Source: three-view drawing plus pictorial views. Frame: mm from the lowest corner of the part. A direction names the side the tool comes from. Give positions to 0.01 mm unless a question says otherwise; leave off trailing zeros. Write each loop counter-clockwise with the first axis right and the second up, starting at its lowest first coordinate (ties: lowest second). Pieces come first, ordered by that corner, then holes.
Q1. Reachability of the marked faces 1 and 2 from +Z, -Z, +X, -X, +Y, -Y: full face, straight path, thin tool, end or side. Return the list, or none.
Q2. Pin query (flat end, axial travel): pin 1 (1 mm diameter, centred on x = 12, z = 11, fed in from -Y); pin 2 (8 mm diameter, centred on x = 16.5, y = 26.5, fed in from +Z). Return the tip coordinate at first contact, or that it passes through.
Q3. Line query: L1, parallel to X at y = 20.5, z = 10.25; L2, parallel to Y at x = 25, z = 1.5; L3, parallel to Z at x = 10.5, y = 47. Output: solid intervals per line, ascending.
Q4. Cut plane D-D on z = 14.5. Return the cut outline in (x, y), plus the area to 3 significant figures.
Q5. Cut plane A-A on y = 9. Return the cut outline in (x, z).
Q6. Draft query along Y for the marked faces 3, 4 and 5. Return one class per face: pulls with the +Y half, pulls with the -Y half, needs draft (parallel to the pull), parting line crosses it, or undercut.
Q7. Cut plane C-C on y = 37. Return the cut outline in (x, z), plus the area to 3 significant figures.
Q8. Cut plane B-B on x = 41. Return the cut outline in (y, z), plus the area to 3 significant figures.
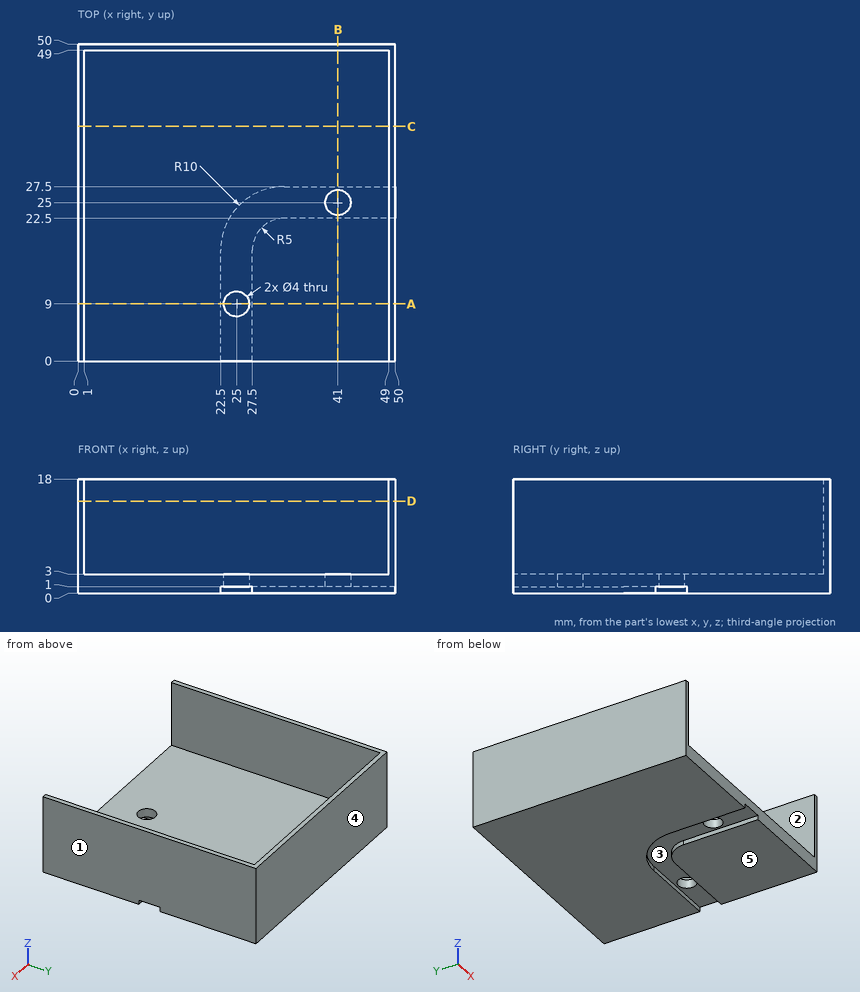
Data:
1. face 1: +Z, -Z, +X, +Y, -Y
1. face 2: +Z, -Y
2. pin 1: stops at y = 49
2. pin 2: stops at z = 3
3. L1: x = 0 to 1, 49 to 50
3. L2: y = 0 to 7, 11 to 50
3. L3: z = 0 to 3
4. outline: (0, 0) - (1, 0) - (1, 49) - (49, 49) - (49, 0) - (50, 0) - (50, 50) - (0, 50) - close
4. area: 148 mm2
5. outline: (0, 0) - (22.5, 0) - (22.5, 1) - (23, 1) - (23, 3) - (1, 3) - (1, 18) - (0, 18) - close; (27, 1) - (27.5, 1) - (27.5, 0) - (50, 0) - (50, 18) - (49, 18) - (49, 3) - (27, 3) - close
6. face 3: undercut
6. face 4: pulls with the +Y half
6. face 5: needs draft
7. outline: (0, 0) - (50, 0) - (50, 18) - (49, 18) - (49, 3) - (1, 3) - (1, 18) - (0, 18) - close
7. area: 180 mm2
8. outline: (0, 0) - (22.5, 0) - (22.5, 1) - (23, 1) - (23, 3) - (0, 3) - close; (27, 1) - (27.5, 1) - (27.5, 0) - (50, 0) - (50, 18) - (49, 18) - (49, 3) - (27, 3) - close
8. area: 152 mm2
